Could you check a few things on this model? Use its own coordinates, in mm. A direction names the side the tool comes from. Round coordinates to 2 decimals unless told otherwise and drop trailing zeros. Write each loop counter-clockwise with the first axis right and the second up, starting at its lowest first coordinate (ties: lowest second). Pieces come first, ordered by that corner, then holes. Notation, with made-up numbers: (-19, 60.25) -> (28, 60.25) arc R14 cw to (28, 65.25) -> close; hole circle Ø11 at (1, 49). An arc over 180 degrees is marked (long way). One line per question, with ' | ' between items. Start each with the question number.
1. For faces 5 (the flat face through (-1, 0, 35)), 6 (the flat face through (-1.4, 3, 1.4)), which set-ups out of +Z, -Z, +X, -X, +Y, -Y let a thin tool reach every point of the face, with its end or its side?
2. Thinking about a two-plate mould opening in X: for faces 1 (the cylindrical face through (-0.1, 3, 75.4)), 2 (the cylindrical face through (0.07, 1.48, 69.8)), 3 (the flat face through (-1, 6, 35)), 4 (the flat face through (-1, 3, 73)), which applies, released by +X, released by -X, zero draft, split by the parting line, or undercut?
3. For pin 1 Ø3 at (x, z) = (1, 0) entering from +Y; pin 2 Ø1.5 at (x, y) = (-3, 3.5) entering from -Z; pin 3 Ø1.5 at (x, y) = (2.5, 4) entering from +Z; pin 4 Ø1.9 at (x, z) = (0, 0) entering from -Y, each with a flat end and sliding along its axis, tell me the tip position at first contact or that it passes through.
4. Imagine slicing it at A-A, the plane x = 0. List the corners of the cut face in (y, z) for me, and give its area (3 significant figures).
5. Imagine slicing it at B-B, the plane y = 1.85. State how many separate pieces and enclosed holes the cut face has, and give its area (3 significant figures).
6. If I drill on line 1 along X through (y, z) = (5.2, 71.4); line 2 along X through (y, z) = (1.9, 71.4); line 3 along Z through (x, y) = (0, 1.15), over which ranges is the centre line in solid material (lowest first)? Write a range as [from, to].
from build123d import *

# Parameters (mm, degrees)
SKETCH_1_R          = 1.6
SKETCH_1_R_2        = 1.6000000000000016
EXTRUDE_1_DEPTH     = 6
CHAMFER_1_SIZE      = 1
SKETCH_2_R          = 3.25
SKETCH_2_R_2        = 3.250000000000001
CUT_EXTRUDE_1_DEPTH = 3


with BuildPart() as part:
    # Эскиз1 → Бобышка-Вытянуть1 (new body)
    with BuildSketch(Plane(origin=(0, 0, 0), x_dir=(1, 0, 0), z_dir=(0, 1, 0))):
        with BuildLine():
            Line((-4, -9.8e-16), (-5.000000000000001, -1.1e-15))
            Line((-5.000000000000001, -1.1e-15), (-4.999999999999991, -71.4))
            Line((-4.999999999999991, -71.4), (-4.000000000000001, -71.4))
            ThreePointArc((-4.000000000000001, -71.4), (-7.3e-16, -75.4), (4, -71.4))
            Line((4, -71.4), (4, 0))
            ThreePointArc((4, 0), (2.4e-16, 4), (-4, -9.8e-16))
        make_face()
        with Locations(Location((0, 0, 0), (0, 0, 270))):
            Circle(SKETCH_1_R, mode=Mode.SUBTRACT)
        with Locations(Location((0, -71.4, 0), (0, 0, 270))):
            Circle(SKETCH_1_R_2, mode=Mode.SUBTRACT)
    extrude(amount=EXTRUDE_1_DEPTH)

    # Фаска1
    chamfer_1_edges = [part.edges().sort_by_distance(p)[0] for p in [
        (-5.000000000000001, 3, 1.1e-15),
        (-4.999999999999991, 3, 71.4),
    ]]
    chamfer(chamfer_1_edges, length=CHAMFER_1_SIZE - 0.0001)  # a hair under: the kernel refuses the full size

    # Эскиз2 → Вырез-Вытянуть1 (cut)
    with BuildSketch(Plane(origin=(0, 6, 0), x_dir=(1, 0, 0), z_dir=(0, 1, 0))):
        with Locations(Location((0, 0, 0), (0, 0, 270))):
            Circle(SKETCH_2_R)
        with Locations(Location((0, -71.4, 0), (0, 0, 270))):
            Circle(SKETCH_2_R_2)
    extrude(amount=-CUT_EXTRUDE_1_DEPTH, mode=Mode.SUBTRACT)


solid = part.part
Geometry results:
1) face 5: +Z, -Z, +X, -X, -Y | face 6: +Y
2) face 1: split by the parting line | face 2: undercut | face 3: zero draft | face 4: undercut
3) pin 1: stops at y = 3 | pin 2: stops at z = -3.31 | pin 3: stops at z = 75 | pin 4: passes through
4) outline: (0, -4) -> (6, -4) -> (6, -3.25) -> (3, -3.25) -> (3, -1.6) -> (0, -1.6) -> close; (0, 1.6) -> (3, 1.6) -> (3, 3.25) -> (6, 3.25) -> (6, 68.15) -> (3, 68.15) -> (3, 69.8) -> (0, 69.8) -> close; (0, 73) -> (3, 73) -> (3, 74.65) -> (6, 74.65) -> (6, 75.4) -> (0, 75.4) -> close | area: 418 mm2
5) separate pieces: 1 | enclosed holes: 2 | area: 676 mm2
6) line 1: x = [-4, -3.25], [3.25, 4] | line 2: x = [-4, -1.6], [1.6, 4] | line 3: z = [-4, -1.6], [1.6, 69.8], [73, 75.4]
